Source: CAD feature listing. Evaluate the final solid. Frame: model axes, mm. A direction names the side the tool comes from. Coordinates: 2 decimals unless noted, no trailing zeros. Write each loop counter-clockwise with the first axis right and the second up, starting at its lowest first coordinate (ties: lowest second). Pieces come first, ordered by that corner, then holes. Notation, with made-up numbers: (40, 23) -> (90, 23) arc R30 cw to (90, 57) -> close; hole circle Ø10 at (-3, 58). An arc over 180 degrees is marked (long way). One line per item, written item: value. Start each with the question number.
1. First-contact query: P1, Ø5, axis at y = 26.67, z = -10.795, coming from the +X side; P2, Ø4, axis at x = 5, z = -3, coming from the +Y side. Flat tips, straight axial feed; report the tip coordinate or a pass-through.
2. Line query: line 1 (Z direction, x = -2.45, y = 11.43) (3 decimals); line 2 (Z direction, x = 2, y = 33) (3 decimals); line 3 (X direction, y = 4, z = -19.75) (3 decimals). Output: solid intervals per line, ascending.
3. Access query for faces 5 (the flat face through (11, 19, 0)), 6 (the cylindrical face through (9.586, 8.598, 1.61)). Directions: +Z, -Z, +X, -X, +Y, -Y. A direction counts if a zero-diameter tool reaches every point of the face in a straight line with its end or side. Return the directions, or none.
4. Mould query, pull axis X, two halves, no side actions, for faces 1 (the flat face through (-3.175, 19, -11)), 2 (the cylindrical face through (-2.74, 13.54, -10.33)), 3 (the cylindrical face through (9.586, 8.598, -23.155)), 4 (the conical face through (-2.143, 13.673, -10.5)). Classes: released by +X, released by -X, zero draft, split by the parting line, or undercut.
5. Section query B-B, the plane y = 16.5. Output: boundary loops of the cut face in (x, z) (3 decimals), and give its area (3 significant figures).
6. Section query C-C, the plane y = 26.67. Output: boundary loops of the cut face in (x, z) (3 decimals).
7. Section query A-A, the plane x = 0.75. Output: boundary loops of the cut face in (y, z) (3 decimals).
8. Section query D-D, the plane z = -1.5. Output: boundary loops of the cut face in (x, y) (3 decimals), and give its area (3 significant figures).
Autodesk Inventor part; units mm, degrees
ref_plane "YZ Plane" through (0, 0, 0) normal (1, 0, 0) x (0, 1, 0)
ref_plane "XZ Plane" through (0, 0, 0) normal (0, 1, 0) x (-1, 0, 0)
ref_plane "XY Plane" through (0, 0, 0) normal (0, 0, 1) x (1, 0, 0)
sketch "Sketch1" plane through (0, 0, 0) normal (0, 1, 0) x (-1, 0, 0)
  line L0 (0, 0) -> (-21.59, 0)
  line L1 (-21.59, 0) -> (-21.59, -21.59)
  line L2 (-21.59, -21.59) -> (0, -21.59)
  line L3 (0, -21.59) -> (0, 0)
  line L4 (-21.59, 0) -> (0, 0)
  line L5 (0, 0) -> (0, 3.175)
  line L6 (0, 3.175) -> (-21.59, 3.175)
  line L7 (-21.59, 3.175) -> (-21.59, 0)
  line L8 (0, 3.175) -> (3.175, 3.175)
  line L9 (3.175, 3.175) -> (3.175, -21.59)
  line L10 (3.175, -21.59) -> (0, -21.59)
  line L11 (0, -21.59) -> (0, 3.175)
  line L12 (3.175, -21.59) -> (-21.59, -21.59)
  line L13 (-21.59, -21.59) -> (-21.59, -24.765)
  line L14 (-21.59, -24.765) -> (3.175, -24.765)
  line L15 (3.175, -24.765) -> (3.175, -21.59)
  dimension "d0" = 21.59
  dimension "d1" = 21.59
  dimension "d2" = 3.175
  dimension "d3" = 3.175
extrude "Extrusion1" add sketch "Sketch1" along normal blind 38.1 contours L5 L8 L9 L10 L3 | L0 L7 L6 L5 | L10 L15 L14 L13 L2
sketch "Sketch2" plane through (0, 0, 0) normal (1, 0, 0) x (0, 0, -1)
  line L0 (0, 0) -> (21.59, 0)
  line L1 (10.795, 0) -> (10.795, 11.43)
  line L2 (10.795, 0) -> (22.225, 0) construction
  line L3 (0, 38.1) -> (21.59, 38.1)
  line L4 (10.795, 38.1) -> (10.795, 26.67)
  line L5 (10.795, 38.1) -> (22.225, 38.1) construction
  circle A0 centre (10.795, 26.67) radius 2.159
  circle A1 centre (10.795, 11.43) radius 2.159
  dimension "d6" = 11.43
  dimension "d7" = 90
  dimension "d8" = 11.43
  dimension "d9" = 90
  dimension "d10" = 15.24
  dimension "d11" = 4.318
  dimension "d12" = 4.318
hole "Hole1" at (0, 26.67, -10.795) at (0, 11.43, -10.795) direction (-1, 0, 0) diameter 4.318 depth 25.4
sketch "Sketch3" plane through (-3.175, 0, 3.175) normal (0, 0, 1) x (1, 0, 0)
  line L0 (3.175, 38.1) -> (24.765, 38.1)
  line L1 (13.97, 38.1) -> (13.97, 28.575)
  circle A0 centre (13.97, 28.575) radius 2.54
  point P0 (3.175, 0)
  dimension "d20" = 9.525
  dimension "d21" = 5.08
extrude "Extrusion2" cut sketch "Sketch3" against normal blind 38.1
sketch "Sketch4" plane through (-3.175, 0, 3.175) normal (0, 0, 1) x (1, 0, 0)
  line L0 (24.765, 0) -> (3.175, 0)
  line L1 (13.97, 0) -> (13.97, 9.525)
  circle A0 centre (13.97, 9.525) radius 1.524
  dimension "d25" = 9.525
  dimension "d26" = 3.048
extrude "Extrusion3" cut sketch "Sketch4" against normal blind 38.1
chamfer "Chamfer1" distance 1.651 distance2 2.286 1 edges at (0, 26.67, -8.636) measured on face at (0, 21.4178, -2.8996)
chamfer "Chamfer2" distance 1.651 distance2 2.286 1 edges at (0, 11.43, -8.636) measured on face at (0, 21.2861, -2.3652)
properties part number "Silder Mount V1"
Computed values:
1. P1: stops at x = -1.81
1. P2: passes through
2. line 1: z = -24.765 to -12.954, -8.636 to 3.175
2. line 2: z = -24.765 to -21.59, 0 to 3.175
2. line 3: x = -3.175 to 0
3. face 5: +X, +Y, -Y
3. face 6: +Z, -Z
4. face 1: released by -X
4. face 2: zero draft
4. face 3: undercut
4. face 4: released by +X
5. outline: (-3.175, -24.765) -> (21.59, -24.765) -> (21.59, -21.59) -> (0, -21.59) -> (0, 0) -> (21.59, 0) -> (21.59, 3.175) -> (-3.175, 3.175) -> close
5. area: 226 mm²
6. outline: (-3.175, -24.765) -> (9.115, -24.765) -> (9.115, -21.59) -> (0, -21.59) -> (0, -14.605) -> (-2.286, -12.954) -> (-3.175, -12.954) -> close; (-3.175, -8.636) -> (-2.286, -8.636) -> (0, -6.985) -> (0, 0) -> (9.115, 0) -> (9.115, 3.175) -> (-3.175, 3.175) -> close; (12.475, -24.765) -> (21.59, -24.765) -> (21.59, -21.59) -> (12.475, -21.59) -> close; (12.475, 0) -> (21.59, 0) -> (21.59, 3.175) -> (12.475, 3.175) -> close
7. outline: (0, -24.765) -> (38.1, -24.765) -> (38.1, -21.59) -> (0, -21.59) -> close; (0, 0) -> (38.1, 0) -> (38.1, 3.175) -> (0, 3.175) -> close
8. outline: (-3.175, 0) -> (0, 0) -> (0, 38.1) -> (-3.175, 38.1) -> close
8. area: 121 mm²
